For this review, take the finished solid that the model builds, in its own axes (mm). A direction names the side the tool comes from. Round coordinates to 2 decimals unless told otherwise and drop trailing zeros. Order: outer loops, then holes, each group sorted by start corner. A loop starts at its lowest first (then second) coordinate and runs counter-clockwise, first axis right, second up. Notation, with made-up numbers: M 47.5,66 L 68.5,66 A14 ccw 68.5,84 Z; hole C 24.25,10 d3. An arc over 180 degrees is marked long. Put each result on its own line as item: value.
from build123d import *

# Parameters (mm, degrees)
F0_W     = 88.9
F0_H     = 25.4
F1_DEPTH = 76.2
F3_DEPTH = 25.4
F4_W     = 25.4
F4_H     = 39.036911
F5_DEPTH = 25.4


with BuildPart() as f1:
    # F0 (on Right) → F1 (new body)
    with BuildSketch(Plane.YZ):
        with Locations((-5.413089, -29.252115)):
            Rectangle(F0_W, F0_H)
    extrude(amount=F1_DEPTH)

    # F2 (on face) → F3 (join)
    with BuildSketch(Plane.XY.offset(-16.552115)):
        Polygon((25.4, 39.036911), (0, 39.036911), (0, 0), (25.4, 0.936911), align=None)
    extrude(amount=F3_DEPTH)

    # F4 (on face) → F5 (join)
    with BuildSketch(Plane.XY.offset(-16.552115)):
        with Locations((63.5, 19.518455)):
            Rectangle(F4_W, F4_H)
    extrude(amount=F5_DEPTH)


solid = f1.part
(1) Add section C-C on y = 19. Give the boundary of the cut face in (x, z).
A:
outline: M 0,-41.95 L 76.2,-41.95 L 76.2,8.85 L 50.8,8.85 L 50.8,-16.55 L 25.4,-16.55 L 25.4,8.85 L 0,8.85 Z
(2) Draft analysis for pull direction X (two halves, no side actions). For faces 4 (the face through (25.4, 20, -4)), 5 (the face through (0, 5, -23)), 6 (the face through (63, 20, 8.848)), state which applies: released by +X, released by -X, zero draft, split by the parting line, or undercut.
A:
face 4: undercut
face 5: released by -X
face 6: zero draft
(3) Add section A-A on z = 4. Give the boundary of the cut face in (x, y).
A:
outline: M 0,0 L 25.4,0.94 L 25.4,39.04 L 0,39.04 Z; M 50.8,0 L 76.2,0 L 76.2,39.04 L 50.8,39.04 Z
(4) To check wall thickness, follow L1, parallel to Y at x = 63, z = -14.5; L2, parallel to Z at x = 9.5, y = -17.5; L3, parallel to Y at x = 18, z = -10. State the ranges of each line that lie inside material, in increasing order.
A:
L1: y = 0 to 39.04
L2: z = -41.95 to -16.55
L3: y = 0.66 to 39.04
(5) Add section B-B on x = 55. Give the boundary of the cut face in (y, z).
A:
outline: M -49.86,-41.95 L 39.04,-41.95 L 39.04,8.85 L 0,8.85 L 0,-16.55 L -49.86,-16.55 Z
(6) Add section D-D on y = -2. Give the boundary of the cut face in (x, z).
A:
outline: M 0,-41.95 L 76.2,-41.95 L 76.2,-16.55 L 0,-16.55 Z
(7) For faces 1 (the face through (50.8, 19, -4)), 2 (the face through (63, 0, -4)), 3 (the face through (12.52, 0.46, -4.03)), list the 3-axis set-ups (+Z, -Z, +X, -X, +Y, -Y) from which the entire face can be reached by the end or side of a thin tool; tool diameter is ignored.
A:
face 1: +Z, +Y, -Y
face 2: +Z, +X, -X, -Y
face 3: +Z, -Y
